Verification items for the finished model (mm, model axes). Face numbers are marked on the shaded views. A direction names the side the tool comes from. Coordinates: 2 decimals unless noted, no trailing zeros. Write each loop counter-clockwise with the first axis right and the second up, starting at its lowest first coordinate (ties: lowest second). Pieces come first, ordered by that corner, then holes.
```python
from build123d import *

# Parameters (mm, degrees)
F0_R     = 15
F0_R_2   = 5
F1_DEPTH = 10
F2_R     = 7.5
F2_R_2   = 5
F3_DEPTH = 5
F4_R     = 12.0112808184
F4_R_2   = 11.2253512915
F4_R_3   = 7.5
F5_DEPTH = 1
F7_DEPTH = 25


with BuildPart() as f1:
    # F0 (on Top) → F1 (new body)
    with BuildSketch(Plane.XY):
        Circle(F0_R)
        Circle(F0_R_2, mode=Mode.SUBTRACT)
    extrude(amount=F1_DEPTH)

    # F2 (on face) → F3 (join)
    with BuildSketch(Plane.XY.offset(10)):
        Circle(F2_R)
        Circle(F2_R_2, mode=Mode.SUBTRACT)
    extrude(amount=F3_DEPTH)

    # F4 (on face) → F5 (cut)
    with BuildSketch(Plane.XY.offset(10)):
        Circle(F4_R)
        Circle(F4_R_2, mode=Mode.SUBTRACT)
        Circle(F4_R_2)
        Circle(F4_R_3, mode=Mode.SUBTRACT)
    extrude(amount=-F5_DEPTH, mode=Mode.SUBTRACT)

    # F6 (on face) → F7 (cut)
    with BuildSketch(Plane.XY.offset(10)):
        Polygon((-1.9454706926, 16.4457075298), (-2.8029684909, 13.6159658432), (1.2272709282, 13.6159658432), (0, 16.4457075298), align=None)
        Polygon((-12.4054077814, -5.7451351204), (-14.242400504, -8.2228537649), (-13.2696651577, -9.907680807), (-10.3902880718, -9.2354248407), align=None)
        Polygon((11.1781368532, -7.8708307228), (14.242400504, -8.2228537649), (15.2151358503, -6.5380267228), (13.1932565627, -4.3805410025), align=None)
    extrude(amount=-F7_DEPTH, mode=Mode.SUBTRACT)


solid = f1.part
```
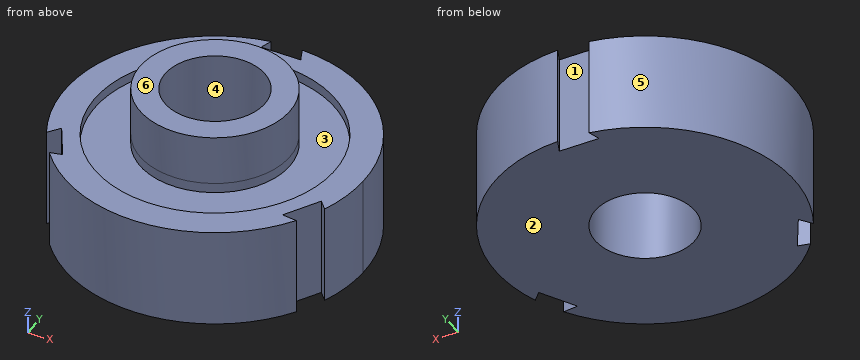
1. Material ranges on L1, parallel to Y at x = 0, z = 9.5; L2, parallel to Y at x = 0, z = 8; L3, parallel to Z at x = -3.5, y = -12.5, recorded low to high.
2. Draft check along Y on the marked faces 4, 5 and 6. Enter one of: pulls with the +Y half, pulls with the -Y half, needs draft (parallel to the pull), parting line crosses it, or undercut.
3. Sectioned sample at C-C, the plane y = -1.5. Record the boundary of the cut face in (x, z), and give its area (3 significant figures).
4. Sectioned sample at A-A, the plane x = 0. Record the boundary of the cut face in (y, z), and give its area (3 significant figures).
5. Sectioned sample at B-B, the plane z = 7. Record the boundary of the cut face in (x, y), and give its area (3 significant figures).
6. Sectioned sample at D-D, the plane x = 9.5. Record the boundary of the cut face in (y, z).
7. Tool access check on the marked faces 1, 2 and 3. Record the directions out of +Z, -Z, +X, -X, +Y, -Y that give a thin tool (end or side, any length) a straight path to the whole face; none if there is none.
8. Gauge pin test, flat ends, axial feed: P1, Ø1, axis at x = 12, z = 9, coming from the +Y side; P2, Ø3, axis at x = 9, y = -11, coming from the +Z side; P3, Ø8, axis at x = -6.5, z = 12, coming from the -Y side. Record the tip position at first contact, or that the pin passes through.
Outcome:
1. L1: y = -15 to -12.01, -7.5 to -5, 5 to 7.5, 12.01 to 13.62
1. L2: y = -15 to -5, 5 to 13.62
1. L3: z = 0 to 10
2. face 4: undercut
2. face 5: parting line crosses it
2. face 6: needs draft
3. outline: (-14.92, 0) - (-4.77, 0) - (-4.77, 15) - (-7.35, 15) - (-7.35, 9) - (-11.92, 9) - (-11.92, 10) - (-14.92, 10) - close; (4.77, 0) - (14.92, 0) - (14.92, 10) - (11.92, 10) - (11.92, 9) - (7.35, 9) - (7.35, 15) - (4.77, 15) - close
3. area: 220 mm2
4. outline: (-15, 0) - (-5, 0) - (-5, 15) - (-7.5, 15) - (-7.5, 9) - (-12.01, 9) - (-12.01, 10) - (-15, 10) - close; (5, 0) - (13.62, 0) - (13.62, 10) - (12.01, 10) - (12.01, 9) - (7.5, 9) - (7.5, 15) - (5, 15) - close
4. area: 202 mm2
5. outline: (-13.3, -6.95) - (-12.41, -5.75) - (-10.39, -9.24) - (-11.59, -9.52) arc R15 ccw to (12.66, -8.04) - (11.18, -7.87) - (13.19, -4.38) - (14.04, -5.28) arc R15 ccw to (0.63, 14.99) - (1.23, 13.62) - (-2.8, 13.62) - (-2.44, 14.8) arc R15 ccw to start; hole circle Ø10 at (0, 0)
5. area: 614 mm2
6. outline: (-11.61, 0) - (11.61, 0) - (11.61, 10) - (7.35, 10) - (7.35, 9) - (-7.35, 9) - (-7.35, 10) - (-11.61, 10) - close
7. face 1: +Z, -Z
7. face 2: -Z, +X, -X, +Y, -Y
7. face 3: +Z
8. P1: stops at y = 9.63
8. P2: stops at z = 10
8. P3: stops at y = -14.69
